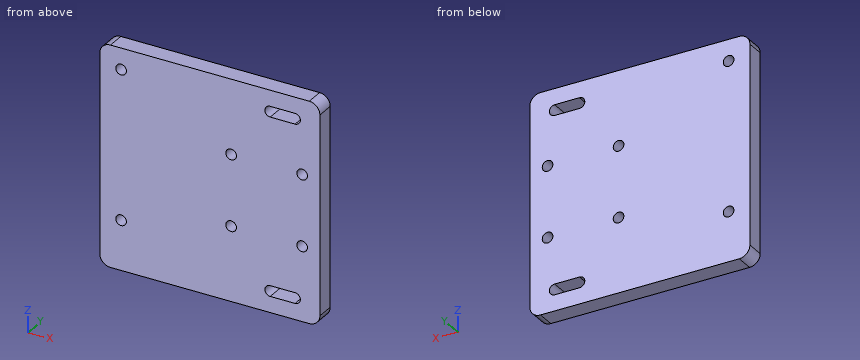
Autodesk Inventor part; units mm, degrees
ref_plane "YZ Plane" through (0, 0, 0) normal (1, 0, 0) x (0, 1, 0)
ref_plane "XZ Plane" through (0, 0, 0) normal (0, 1, 0) x (-1, 0, 0)
ref_plane "XY Plane" through (0, 0, 0) normal (0, 0, 1) x (1, 0, 0)
sketch "Sketch1" plane through (0, 0, 0) normal (0, 1, 0) x (-1, 0, 0)
  line L0 (0, 0) -> (46, 0) construction
  line L1 (46, 0) -> (46, -46) construction
  line L2 (46, -46) -> (0, -46) construction
  line L3 (0, -46) -> (0, 0) construction
  circle A0 centre (46, -46) radius 1.5
  circle A1 centre (46, 0) radius 1.5
  circle A2 centre (0, 0) radius 1.5
  circle A3 centre (0, -46) radius 1.5
  line L4 (23, 0) -> (23, -46) construction
  line L5 (-8, 8) -> (54, 8)
  line L6 (54, 8) -> (54, -54)
  line L7 (54, -54) -> (-8, -54)
  line L8 (-8, -54) -> (-8, 8)
  line L9 (-8, 8) -> (54, -54) construction
  line L10 (54, 8) -> (-8, -54) construction
  point P0 (23, -23)
  dimension "d0" = 46
  dimension "d1" = 46
  dimension "d2" = 3
  dimension "d3" = 3
  dimension "d4" = 3
  dimension "d5" = 3
  dimension "d6" = 8
  dimension "d7" = 8
extrude "Extrusion1" add sketch "Sketch1" along normal blind 5
sketch "Sketch2" plane through (0, 5, 0) normal (0, 1, 0) x (1, 0, 0)
  line L0 (-54, -8) -> (8, -8)
  line L1 (-54, -8) -> (-114, -8)
  line L2 (-114, -8) -> (-114, 54)
  line L3 (-114, 54) -> (-54, 54)
  line L4 (-54, 54) -> (-54, -8)
  line L5 (8, 54) -> (-54, 54)
  point P0 (0, 0)
  dimension "d10" = 60
extrude "Extrusion2" add sketch "Sketch2" against normal blind 5
sketch "Sketch3" plane through (0, 5, 0) normal (0, 1, 0) x (1, 0, 0)
  circle A0 centre (0, 46) radius 1.5
  circle A1 centre (-46, 46) radius 1.5
  line L0 (0, 46) -> (-46, 46) construction
  line L1 (-23, 46) -> (-23, 0) construction
  line L2 (-1.5, 44.5) -> (-44.5, 44.5)
  line L3 (-44.5, 44.5) -> (-44.5, 1.5)
  line L4 (-44.5, 1.5) -> (-1.5, 1.5)
  line L5 (-1.5, 1.5) -> (-1.5, 44.5)
  line L6 (-1.5, 44.5) -> (-44.5, 1.5) construction
  line L7 (-44.5, 44.5) -> (-1.5, 1.5) construction
  line L8 (-114, -8) -> (8, -8)
  point P0 (0, 0)
  point P1 (-23, 23)
  dimension "d14" = 43
  dimension "d15" = 43
extrude "Extrusion3" cut sketch "Sketch3" against normal blind 5 contours L5 L4 L3 L2
fillet "Fillet1" radius 1 4 edges at (-44.5, 2.5, -44.5) (-44.5, 2.5, -1.5) (-1.5, 2.5, -1.5) (-1.5, 2.5, -44.5)
sketch "Sketch4" plane through (0, 5, 0) normal (0, 1, 0) x (1, 0, 0)
  circle A0 centre (-108, 40) radius 1.5
  circle A1 centre (-108, -2) radius 1.5
  line L0 (-114, -8) -> (8, -8)
  line L1 (-114, 54) -> (-114, -8)
  line L2 (8, 54) -> (-114, 54)
  circle A2 centre (-59, -2) radius 1.5
  circle A3 centre (-59, 48) radius 1.5
  circle A4 centre (-66, -2) radius 1.5
  circle A5 centre (-66, 48) radius 1.5
  line L3 (-59, -2) -> (-59, 48) construction
  line L4 (-66, 46.5) -> (-59, 46.5)
  line L5 (-66, 49.5) -> (-59, 49.5)
  line L6 (-66, -3.5) -> (-59, -3.5)
  line L7 (-66, -0.5) -> (-59, -0.5)
  line L8 (-66, -2) -> (-66, 48) construction
  line L9 (-59, -2) -> (-66, -2) construction
  line L10 (-59, 48) -> (-66, 48) construction
  point P0 (0, 0)
  dimension "d19" = 6
  dimension "d20" = 3
  dimension "d21" = 6
  dimension "d23" = 3
  dimension "d24" = 6
  dimension "d25" = 14
  dimension "d26" = 3
  dimension "d27" = 3
  dimension "d28" = 50
  dimension "d29" = 6
  dimension "d32" = 7
  dimension "d33" = 3
  dimension "d34" = 3
  dimension "d35" = 7
  dimension "d36" = 42
extrude "Extrusion4" cut sketch "Sketch4" against normal blind 5
fillet "Fillet2" radius 3 4 edges at (8, 2.5, -54) (8, 2.5, 8) (-114, 2.5, 8) (-114, 2.5, -54)
sketch "Sketch5" plane through (0, 5, 0) normal (0, 1, 0) x (1, 0, 0)
  line L0 (-52, 54) -> (8, 54)
  line L1 (8, 54) -> (8, -8)
  line L2 (8, -8) -> (-52, -8)
  line L3 (-52, -8) -> (-52, 54)
  point P0 (0, 0)
extrude "Extrusion5" cut sketch "Sketch5" against normal blind 10
fillet "Fillet3" radius 3 2 edges at (-52, 2.5, 8) (-52, 2.5, -54)
sketch "Sketch6" plane through (0, 5, 0) normal (0, 1, 0) x (1, 0, 0)
  line L0 (-52, 51) -> (-52, -5)
  line L1 (-52, 23) -> (-67, 23) construction
  line L2 (-77, 33) -> (-57, 33) construction
  line L3 (-57, 33) -> (-57, 13) construction
  line L4 (-57, 13) -> (-77, 13) construction
  line L5 (-77, 13) -> (-77, 33) construction
  line L6 (-77, 33) -> (-57, 13) construction
  line L7 (-57, 33) -> (-77, 13) construction
  circle A0 centre (-57, 33) radius 1.5
  circle A1 centre (-57, 13) radius 1.5
  circle A2 centre (-77, 13) radius 1.5
  circle A3 centre (-77, 33) radius 1.5
  point P0 (0, 0)
  dimension "d44" = 20
  dimension "d45" = 20
  dimension "d46" = 5
  dimension "d47" = 3
  dimension "d48" = 3
  dimension "d49" = 3
  dimension "d50" = 3
extrude "Extrusion6" cut sketch "Sketch6" against normal blind 10
properties part number "Electronics base"
Build history of the part. All positions in model axes, mm. Round coordinates to 2 decimals unless told otherwise and drop trailing zeros. Loops run counter-clockwise (first coordinate to the right, second up) from the corner with the lowest first, then second, coordinate; pieces in that order, holes last.
Item 1: Saw through at C-C (z = -48). List the corners of the cut face in (x, y), then the cut area to 3 significant figures.
Item 2: Saw through at B-B (x = -64). List the corners of the cut face in (y, z), then the cut area to 3 significant figures.
Item 3: Saw through at D-D (y = 3.45). State how many separate pieces and enclosed holes the cut face has, then the cut area to 3 significant figures.
Item 4: Drill centre lines: line 1 along X through (y, z) = (3.4, -33); line 2 along X through (y, z) = (2.8, 2); line 3 along Z through (x, y) = (-77, 2.5). Where is each one in solid material? Low to high.
Item 5: Pin check, flat tip, straight feed: P1, Ø2.5, axis at x = -108, z = -40, coming from the +Y side. Stop position of the tip, or through.
Item 6: Saw through at A-A (z = -13). List the corners of the cut face in (x, y), then the cut area to 3 significant figures.
Worked answers:
1. outline: (-114, 0) - (-67.5, 0) - (-67.5, 5) - (-114, 5) - close; (-57.5, 0) - (-52, 0) - (-52, 5) - (-57.5, 5) - close
1. area: 260 mm2
2. outline: (0, -54) - (5, -54) - (5, -49.5) - (0, -49.5) - close; (0, -46.5) - (5, -46.5) - (5, 0.5) - (0, 0.5) - close; (0, 3.5) - (5, 3.5) - (5, 8) - (0, 8) - close
2. area: 280 mm2
3. separate pieces: 1
3. enclosed holes: 8
3. area: 3,740 mm2
4. line 1: x = -114 to -78.5, -75.5 to -58.5, -55.5 to -52
4. line 2: x = -114 to -109.5, -106.5 to -67.5, -57.5 to -52
4. line 3: z = -54 to -34.5, -31.5 to -14.5, -11.5 to 8
5. P1: passes through
6. outline: (-114, 0) - (-78.5, 0) - (-78.5, 5) - (-114, 5) - close; (-75.5, 0) - (-58.5, 0) - (-58.5, 5) - (-75.5, 5) - close; (-55.5, 0) - (-52, 0) - (-52, 5) - (-55.5, 5) - close
6. area: 280 mm2
